```python
from build123d import *

# Parameters (mm, degrees)
BOSS_EXTRUDE1_DEPTH     = 40.64
BOSS_EXTRUDE2_DEPTH     = 40.64
SKETCH3_W               = 101.6
SKETCH3_H               = 106.68
BOSS_EXTRUDE3_DEPTH     = 71.12
CUT_EXTRUDE1_DEPTH      = 260.875641029
CUT_EXTRUDE1_DEPTH_BACK = 260.875641029
SKETCH5_W               = 101.6
SKETCH5_H               = 30.48
BOSS_EXTRUDE4_DEPTH     = 71.12
CUT_EXTRUDE2_DEPTH      = 71.12


with BuildPart() as part:
    # Sketch1 → Boss-Extrude1 (new body)
    with BuildSketch(Plane(origin=(0, 0, 0), x_dir=(1, 0, 0), z_dir=(0, 1, 0))):
        with BuildLine():
            Line((-121.92, -81.28), (121.92, -81.28))
            Line((121.92, -81.28), (121.92, -20.32))
            Line((121.92, -20.32), (71.12, -20.32))
            ThreePointArc((71.12, -20.32), (50.8, 0), (71.12, 20.32))
            Line((71.12, 20.32), (121.92, 20.32))
            Line((121.92, 20.32), (121.92, 81.28))
            Line((121.92, 81.28), (-121.92, 81.28))
            Line((-121.92, 81.28), (-121.92, -81.28))
        make_face()
    extrude(amount=BOSS_EXTRUDE1_DEPTH)

    # Sketch2 → Boss-Extrude2 (add)
    with BuildSketch(Plane.ZY.offset(121.92)):
        with BuildLine():
            Line((-81.28, 40.64), (-81.28, 203.2))
            ThreePointArc((-81.28, 203.2), (33.66727835, 155.58727835), (81.28, 40.64))
            Line((81.28, 40.64), (-81.28, 40.64))
        make_face()
    extrude(amount=-BOSS_EXTRUDE2_DEPTH)

    # Sketch3 → Boss-Extrude3 (add)
    with BuildSketch(Plane(origin=(0, 40.64, 0), x_dir=(1, 0, 0), z_dir=(0, 1, 0))):
        with Locations((-30.48, 27.94)):
            Rectangle(SKETCH3_W, SKETCH3_H)
    extrude(amount=BOSS_EXTRUDE3_DEPTH)

    # Sketch4 → Cut-Extrude1 (cut, two sides: drawn at the far end of the back side and taken through both)
    with BuildSketch(Plane.XY.offset(25.4).offset(-CUT_EXTRUDE1_DEPTH_BACK)):
        with BuildLine():
            Line((-60.96, 111.76), (0, 111.76))
            ThreePointArc((0, 111.76), (-30.48, 81.28), (-60.96, 111.76))
        make_face()
    extrude(amount=CUT_EXTRUDE1_DEPTH + CUT_EXTRUDE1_DEPTH_BACK, mode=Mode.SUBTRACT)

    # Sketch5 → Boss-Extrude4 (add)
    with BuildSketch(Plane(origin=(0, 40.64, 0), x_dir=(1, 0, 0), z_dir=(0, 1, 0))):
        with Locations((71.12, 66.04)):
            Rectangle(SKETCH5_W, SKETCH5_H)
    extrude(amount=BOSS_EXTRUDE4_DEPTH)

    # Sketch6 → Cut-Extrude2 (cut)
    with BuildSketch(Plane.XY.offset(-50.8)):
        Polygon((20.32, 111.76), (121.92, 40.64), (121.92, 111.76), align=None)
    extrude(amount=-CUT_EXTRUDE2_DEPTH, mode=Mode.SUBTRACT)


solid = part.part
```
Could you check a few things on this model? Use its own coordinates, in mm. A direction names the side the tool comes from. Give positions to 0.01 mm unless a question says otherwise; leave off trailing zeros. Loops run counter-clockwise (first coordinate to the right, second up) from the corner with the lowest first, then second, coordinate; pieces in that order, holes last. Notation, with made-up numbers: (-9, 15.25) - (48, 15.25) arc R17 ccw to (48, 33.25) - close; hole circle Ø10 at (37.5, 4.5). An arc over 180 degrees is marked (long way). Answer in a Markdown table with one row per item. Add a question column.
Q1. For pin 1 (21.5 mm diameter, centred on x = 47.5, y = 71, fed in from +Z); pin 2 (4 mm diameter, centred on x = -78, z = 9.5, fed in from +Y); pin 3 (12 mm diameter, centred on x = -20.5, z = -11.5, fed in from +Y), each with a flat end and sliding along its axis, tell me the tip position at first contact or that it passes through.
Q2. Please list where these lines run through material, in increasing order: L1, parallel to X at y = 110, z = 7.5; L2, parallel to Z at x = -46, y = 80; L3, parallel to Y at x = 28, z = 70. Write a range as from..to.
Q3. If we section it at A-A (x = 94): List the corners of the cut face in (y, z) for me, plus the area to 3 significant figures.
Q4. If we section it at D-D (x = -11): List the corners of the cut face in (y, z) for me, plus the area to 3 significant figures.
Q5. We'd pull the mould along Z, two halves only. Please class faces 5 (the face through (96, 20, -20.32)), 6 (the face through (-29, 78, -81.28)), 7 (the face through (121.92, 20, -50)), 8 (the face through (-2, 20, 81.28)): +Z half, -Z half, draft (parallel to the pull), parting line (faces both ways), or undercut.
Q6. If we section it at B-B (y = 47): List the corners of the cut face in (x, z) for me, plus the area to 3 significant figures.
Q7. If we section it at C-C (z = -10): List the corners of the cut face in (x, y) for me, plus the area to 3 significant figures.
Q8. Which directions (+Z, -Z, +X, -X, +Y, -Y) give clear straight access to the entire face, cutting with the end or side of a thin tool? Please do faces 1 (the face through (10, 111.76, -29)), 2 (the face through (59, 68, -50.8)), 3 (the face through (-2, 0, -1)), 4 (the face through (97, 20, 20.32)).
The answers:
| question | item | result |
|---|---|---|
| 1 | pin 1 | stops at z = -50.8 |
| 1 | pin 2 | stops at y = 111.76 |
| 1 | pin 3 | stops at y = 85.8 |
| 2 | L1 | x = -121.92..-60.91, -0.05..20.32 |
| 2 | L2 | z = -81.28..25.4 |
| 2 | L3 | y = 0..40.64 |
| 3 | outline | (0, -81.28) - (60.18, -81.28) - (60.18, -50.8) - (40.64, -50.8) - (40.64, -20.32) - (0, -20.32) - close; (0, 20.32) - (40.64, 20.32) - (40.64, 81.28) - (0, 81.28) - close |
| 3 | area | 5,550 mm^2 |
| 4 | outline | (0, -81.28) - (88.32, -81.28) - (88.32, 25.4) - (40.64, 25.4) - (40.64, 81.28) - (0, 81.28) - close |
| 4 | area | 11,700 mm^2 |
| 5 | face 5 | undercut |
| 5 | face 6 | -Z half |
| 5 | face 7 | draft |
| 5 | face 8 | +Z half |
| 6 | outline | (-121.92, -81.28) - (112.83, -81.28) - (112.83, -50.8) - (20.32, -50.8) - (20.32, 25.4) - (-81.28, 25.4) - (-81.28, 81.16) - (-121.92, 81.16) - close |
| 6 | area | 20,300 mm^2 |
| 7 | outline | (-121.92, 0) - (53.43, 0) - (53.43, 40.64) - (20.32, 40.64) - (20.32, 111.76) - (0, 111.76) arc R30.48 cw to (-60.96, 111.76) - (-81.28, 111.76) - (-81.28, 186.74) - (-121.92, 186.74) - close |
| 7 | area | 18,800 mm^2 |
| 8 | face 1 | +Z, -Z, +X, +Y |
| 8 | face 2 | +Z, +X, +Y |
| 8 | face 3 | +Z, -Z, +X, -X, -Y |
| 8 | face 4 | +X, +Y, -Y |
